Geometry: final body of the model. Coordinates: model frame, mm. Face numbers are marked on the shaded views. A direction names the side the tool comes from. Round coordinates to 2 decimals unless told otherwise and drop trailing zeros. Loops run counter-clockwise (first coordinate to the right, second up) from the corner with the lowest first, then second, coordinate; pieces in that order, holes last. Notation, with made-up numbers: (52.25, 73.5) - (62.25, 73.5) arc R21 ccw to (62.25, 107.5) - close; hole circle Ø7 at (72.25, 55). An arc over 180 degrees is marked (long way). Return JSON: item names as keys, results as strings. Group by question number.
1. Section C-C on y = -7.5. Return loops of the section in (x, z), and give its area (3 significant figures).
2. Draft query along Y for the marked faces 3, 4 and 5. Return one class per face: +Y half, -Y half, draft (parallel to the pull), parting line (faces both ways), or undercut.
3. First-contact query: pin 1 Ø1 at (x, y) = (48, -1) entering from +Z; pin 2 Ø6 at (y, z) = (-22, 36.5) entering from -X. Flat tips, straight axial feed; report the tip coordinate or a pass-through.
4. Section A-A on x = 33.25. Return loops of the section in (y, z).
5. Section B-B on z = 36. Return loops of the section in (x, y).
6. Material intervals for probe 1 along X at (y, z) = (-5, 23.65); probe 2 along Y at (x, z) = (52, 30.5); probe 3 along Y at (x, z) = (33.25, 24.05), sorted ascending.
7. Section D-D on x = 47. Return loops of the section in (y, z), and give its area (3 significant figures).
8. Set-up query: the marked faces 1 and 2. Return all of +Z, -Z, +X, -X, +Y, -Y with unobstructed straight access to the full face (end or side cutting, diameter ignored); none if empty.
from build123d import *

# Parameters (mm, degrees)
SKETCH026_W           = 57.3
SKETCH026_H           = 49.2
SKETCH026_R           = 1.6
PAD010002001016_DEPTH = 16.5
FILLET004_R           = 7.3
SKETCH028_W           = 53.6778
SKETCH028_H           = 32.7182
POCKET001_DEPTH       = 14


with BuildPart() as part:
    # Sketch026 → Pad010002001016 (new body)
    with BuildSketch(Plane(origin=(48, -5, 22), x_dir=(0, 1, 0), z_dir=(0, 0, 1))):
        Rectangle(SKETCH026_W, SKETCH026_H)
        with Locations((0, 14.75)):
            Circle(SKETCH026_R, mode=Mode.SUBTRACT)
        with Locations((0, -14.75)):
            Circle(SKETCH026_R, mode=Mode.SUBTRACT)
    extrude(amount=PAD010002001016_DEPTH)

    # Fillet004
    fillet004_edges = [part.edges().sort_by_distance(p)[0] for p in [
        (72.6, -5, 38.5),
        (23.4, -5, 38.5),
    ]]
    fillet(fillet004_edges, radius=FILLET004_R)

    # Sketch028 → Pocket001 (cut)
    with BuildSketch(Plane(origin=(48, -5, 38.5), x_dir=(0, 1, 0), z_dir=(0, 0, 1))):
        Rectangle(SKETCH028_W, SKETCH028_H)
    extrude(amount=-POCKET001_DEPTH, mode=Mode.SUBTRACT)


solid = part.part
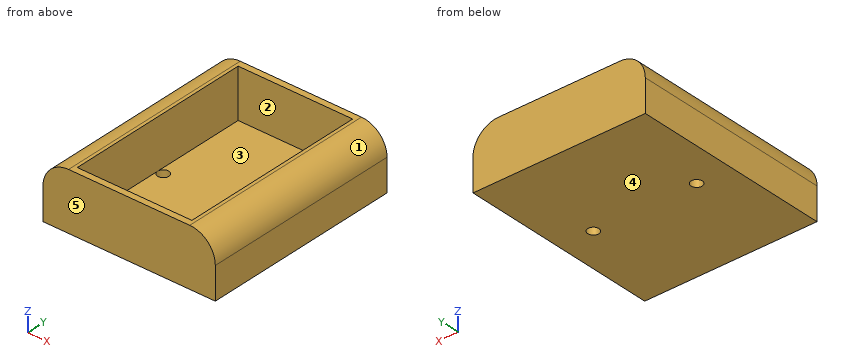
Taken from the geometry:
{
 "1": {"outline": "(23.4, 22) - (72.6, 22) - (72.6, 31.2) arc R7.3 ccw to (65.3, 38.5) - (64.36, 38.5) - (64.36, 24.5) - (31.64, 24.5) - (31.64, 38.5) - (30.7, 38.5) arc R7.3 ccw to (23.4, 31.2) - close", "area": "331 mm2"},
 "2": {"face 3": "undercut", "face 4": "draft", "face 5": "-Y half"},
 "3": {"pin 1": "z = 24.5", "pin 2": "x = 23.77"},
 "4": {"outline": "(-33.65, 22) - (-6.6, 22) - (-6.6, 24.5) - (-31.84, 24.5) - (-31.84, 38.5) - (-33.65, 38.5) - close; (-3.4, 22) - (23.65, 22) - (23.65, 38.5) - (21.84, 38.5) - (21.84, 24.5) - (-3.4, 24.5) - close"},
 "5": {"outline": "(25.2, -33.65) - (70.8, -33.65) - (70.8, 23.65) - (25.2, 23.65) - close; hole (31.64, -31.84) - (64.36, -31.84) - (64.36, 21.84) - (31.64, 21.84) - close"},
 "6": {"probe 1": "23.4 to 31.65, 34.85 to 61.15, 64.35 to 72.6", "probe 2": "-33.65 to -31.84, 21.84 to 23.65", "probe 3": "-33.65 to -6.6, -3.4 to 23.65"},
 "7": {"outline": "(-33.65, 22) - (23.65, 22) - (23.65, 38.5) - (21.84, 38.5) - (21.84, 24.5) - (-31.84, 24.5) - (-31.84, 38.5) - (-33.65, 38.5) - close", "area": "194 mm2"},
 "8": {"face 1": "+Z, +X, +Y, -Y", "face 2": "+Z"}
}
